Build history of the part. All positions in model axes, mm. Face numbers are marked on the shaded views. Coordinates: 2 decimals unless noted, no trailing zeros. Order: outer loops, then holes, each group sorted by start corner. A loop starts at its lowest first (then second) coordinate and runs counter-clockwise, first axis right, second up. Notation, with made-up numbers: (67.25, 48.25) - (108.25, 48.25) arc R26 ccw to (108.25, 74.25) - close; hole circle Ø6 at (-14.75, 51). An arc over 180 degrees is marked (long way). Return JSON: item names as keys, results as strings.
from build123d import *

# Parameters (mm, degrees)
F0_R     = 15
F0_R_2   = 13
F1_DEPTH = 100
F5_W     = 78.4293748438
F5_H     = 68.3440808207
F6_DEPTH = 25
F8_W     = 147.4837362766
F8_H     = 68.2909283787
F9_DEPTH = 35


with BuildPart() as f1:
    # F0 (on Front) → F1 (new body)
    with BuildSketch(Plane.XZ):
        Circle(F0_R)
        Circle(F0_R_2, mode=Mode.SUBTRACT)
    extrude(amount=F1_DEPTH)

    # F5 (on offset) → F6 (cut)
    with BuildSketch(Plane(origin=(-0.1664731949, -10.0254920816, 10.0241098435), x_dir=(0.9999310662, -0.0083030673, 0.0083019226), z_dir=(-0.011741501, -0.7071067812, 0.7070092907))):
        with Locations((-2.7506519109, -14.8982955143)):
            Rectangle(F5_W, F5_H)
    extrude(amount=-F6_DEPTH, mode=Mode.SUBTRACT)

    # F8 (on offset) → F9 (cut)
    with BuildSketch(Plane(origin=(-0.5816526691, -35.0287878644, 35.0239583631), x_dir=(0.9999310662, -0.0083030673, 0.0083019226), z_dir=(-0.011741501, -0.7071067812, 0.7070092907))):
        with Locations((9.9375471473, -57.1080548689)):
            Rectangle(F8_W, F8_H)
    extrude(amount=F9_DEPTH, mode=Mode.SUBTRACT)


solid = f1.part
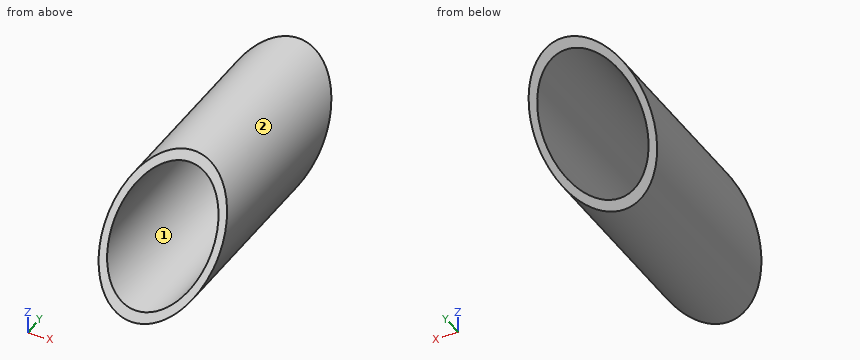
1. Cut at D-D on y = -66. Give the cut face in (x, z), plus the area to 3 significant figures.
Check values:
{"outline": "(-14.51, 3.82) arc R15 ccw (long way) to (14.37, 4.3) - (12.28, 4.26) arc R13 cw (long way) to (-12.42, 3.85) - close", "area": "104 mm²"}
2. Probe L1, parallel to Z at x = 0, y = -55; L2, parallel to X at y = -72, z = -9.25; L3, parallel to X at y = -50, z = 1.25. List the from-to ranges inside material, lowest first.
Check values:
{"L1": "-15 to -13, 13 to 15", "L2": "-11.81 to -9.13, 9.13 to 11.81", "L3": "-14.95 to -12.94, 12.94 to 14.95"}
3. Cut at C-C on y = -44. Give the cut face in (x, z).
Check values:
{"outline": "circle Ø30 at (0, 0); hole circle Ø26 at (0, 0)"}
4. Cut at A-A on z = 4.75. Give the cut face in (x, y), plus the area to 3 significant figures.
Check values:
{"outline": "(-14.23, -65.07) - (-12.1, -65.11) - (-12.1, -15.1) - (-14.23, -15.07) - close; (12.1, -65.51) - (14.23, -65.54) - (14.23, -15.54) - (12.1, -15.5) - close", "area": "213 mm²"}
5. Mould opens along Z. For the marked faces 1 and 2 say: pulls with the +Z half, pulls with the -Z half, needs draft (parallel to the pull), parting line crosses it, or undercut.
Check values:
{"face 1": "undercut", "face 2": "parting line crosses it"}
6. Cut at B-B on x = 6.5. Give the cut face in (y, z).
Check values:
{"outline": "(-83.68, -13.52) - (-33.68, -13.52) - (-31.42, -11.26) - (-81.42, -11.26) - close; (-58.91, 11.26) - (-8.9, 11.26) - (-6.64, 13.52) - (-56.65, 13.52) - close"}
7. Drop flat-ended pins along their axis: pin 1 (2 mm diameter, centred on x = 12, z = -9, fed in from +Y); pin 2 (10 mm diameter, centred on x = -0.5, y = -14.5, fed in from -Z); pin 3 (6 mm diameter, centred on y = -61.5, z = 10, fed in from -X). Give the stop position or say it passes through.
Check values:
{"pin 1": "y = -28.25", "pin 2": "z = 11.78", "pin 3": "x = -13.27"}
